Input: part model. Units: mm. Frame: model coordinates. Face numbers are marked on the shaded views. A direction names the side the tool comes from. Round coordinates to 2 decimals unless told otherwise and drop trailing zeros. Loops run counter-clockwise (first coordinate to the right, second up) from the corner with the lowest first, then second, coordinate; pieces in that order, holes last.
(1) Access query for the marked faces 1 and 2. Directions: +Z, -Z, +X, -X, +Y, -Y. A direction counts if a zero-diameter tool reaches every point of the face in a straight line with its end or side. Return the directions, or none.
(2) Cut plane B-B, the plane x = 5. Give the number of separate pieces and of enclosed holes in the cut face, and give its area (3 significant figures).
(3) Cut plane D-D, the plane y = 26.5. Output: boundary loops of the cut face in (x, z), and give its area (3 significant figures).
(4) Draft query along Y for the marked faces 3, 4 and 5. Return one class per face: released by +Y, released by -Y, zero draft, split by the parting line, or undercut.
(5) Cut plane A-A, the plane y = 13. Output: boundary loops of the cut face in (x, z), and give its area (3 significant figures).
(6) Cut plane C-C, the plane z = 2.75. Output: boundary loops of the cut face in (x, y), and give its area (3 significant figures).
(7) Line query: line 1 (Y direction, x = 5, z = 2); line 2 (Y direction, x = 5.5, z = 5); line 3 (Y direction, x = 2.75, z = 3.25) (3 decimals). Output: solid intervals per line, ascending.
(8) First-contact query: pin 1 Ø1.5 at (x, y) = (7, 26.5) entering from -Z; pin 2 Ø4.5 at (x, y) = (5, 15) entering from +Z. Flat tips, straight axial feed; report the tip coordinate or a pass-through.
from build123d import *

# Parameters (mm, degrees)
SKETCH1_W               = 10
SKETCH1_H               = 20
BOSS_EXTRUDE1_DEPTH     = 7
SKETCH2_R               = 3.5
BOSS_EXTRUDE2_DEPTH     = 15
SKETCH3_R               = 2.5
CUT_EXTRUDE1_DEPTH      = 38.067505986
CUT_EXTRUDE2_DEPTH      = 37.961317978
CUT_EXTRUDE2_DEPTH_BACK = 37.961317978
CHAMFER1_SIZE           = 2
CHAMFER2_SIZE           = 1


with BuildPart() as part:
    # Sketch1 → Boss-Extrude1 (new body)
    with BuildSketch(Plane.XY):
        with Locations((5, 10)):
            Rectangle(SKETCH1_W, SKETCH1_H)
    extrude(amount=BOSS_EXTRUDE1_DEPTH)

    # Sketch2 → Boss-Extrude2 (add)
    with BuildSketch(Plane(origin=(0, 20, 0), x_dir=(1, 0, 0), z_dir=(0, 1, 0))):
        with Locations(Location((4.5, -3.5, 0), (0, 0, 90))):
            Circle(SKETCH2_R)
    extrude(amount=BOSS_EXTRUDE2_DEPTH)

    # Sketch3 → Cut-Extrude1 (cut, through all)
    with BuildSketch(Plane.XY.offset(7)):
        with Locations((5, 15)):
            Circle(SKETCH3_R)
        with Locations((5, 5)):
            Circle(SKETCH3_R)
    extrude(amount=-CUT_EXTRUDE1_DEPTH, mode=Mode.SUBTRACT)

    # Sketch4 → Cut-Extrude2 (cut, two sides: drawn at the far end of the back side and taken through both)
    with BuildSketch(Plane(origin=(-0.597969362, 0, 1.631380802), x_dir=(0.9389141835786157, 0, 0.34415135605559033), z_dir=(-0.34415135605559033, 0, 0.9389141835786157)).offset(-CUT_EXTRUDE2_DEPTH_BACK)):
        Polygon((1.929643572, 35), (3.419643572, 35), (3.419643572, 34.4), (3.919643572, 34.4), (3.919643572, 33.4), (1.929643572, 31.265986267), align=None)
    extrude(amount=CUT_EXTRUDE2_DEPTH + CUT_EXTRUDE2_DEPTH_BACK, mode=Mode.SUBTRACT)

    # Chamfer1
    chamfer1_edges = [part.edges().sort_by_distance(p)[0] for p in [
        (10, 20, 3.5),
        (10, 0, 3.5),
        (0, 0, 3.5),
    ]]
    chamfer(chamfer1_edges, length=CHAMFER1_SIZE - 0.0001)  # a hair under: the kernel refuses the full size

    # Chamfer2
    chamfer2_edges = [part.edges().sort_by_distance(p)[0] for p in [
        (0, 20, 3.5),
    ]]
    chamfer(chamfer2_edges, length=CHAMFER2_SIZE - 0.0001)  # a hair under: the kernel refuses the full size


solid = part.part
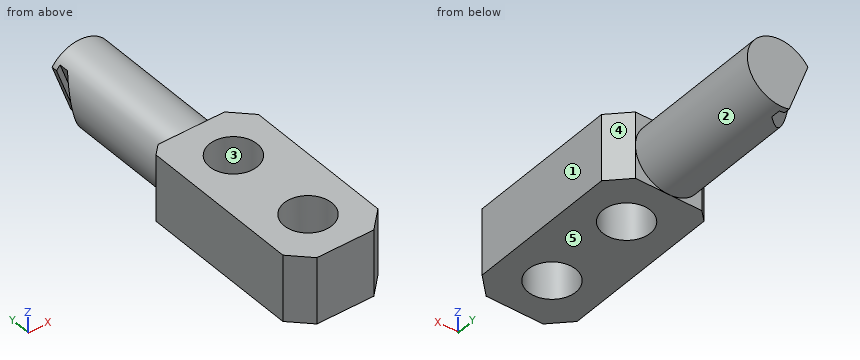
Reported:
1. face 1: +Z, -Z, +X, +Y, -Y
1. face 2: +Y
2. separate pieces: 3
2. enclosed holes: 0
2. area: 174 mm2
3. outline: circle Ø7 at (4.5, 3.5)
3. area: 38.5 mm2
4. face 3: undercut
4. face 4: released by +Y
4. face 5: zero draft
5. outline: (0, 0) - (3.5, 0) - (3.5, 7) - (0, 7) - close; (6.5, 0) - (10, 0) - (10, 7) - (6.5, 7) - close
5. area: 49.0 mm2
6. outline: (0, 2) - (2, 0) - (8, 0) - (10, 2) - (10, 18) - (8, 20) - (7.92, 20) - (7.92, 35) - (2.63, 35) - (2.63, 34.4) - (3.17, 34.4) - (3.17, 33.4) - (1.08, 31.3) - (1.08, 20) - (1, 20) - (0, 19) - close; hole circle Ø5 at (5, 5); hole circle Ø5 at (5, 15)
6. area: 252 mm2
7. line 1: y = 0 to 2.5, 7.5 to 12.5, 17.5 to 35
7. line 2: y = 0 to 2.55, 7.45 to 12.55, 17.45 to 35
7. line 3: y = 0 to 3.91, 6.09 to 13.91, 16.09 to 33.165, 34.4 to 35
8. pin 1: stops at z = 0.47
8. pin 2: passes through
